Job drawing, mm, ordinate dimensions from the low corner. One solid piece. Give positions to 0.01 mm unless a question says otherwise; leave off trailing zeros. Loops run counter-clockwise (first coordinate to the right, second up) from the corner with the lowest first, then second, coordinate; pieces in that order, holes last. Notation, with made-up numbers: M 16,-6 L 29,-6 A20 cw 29,8 Z; hole C 14.25,54 d2. An arc over 180 degrees is marked long. Answer in a Markdown table with one row per item.
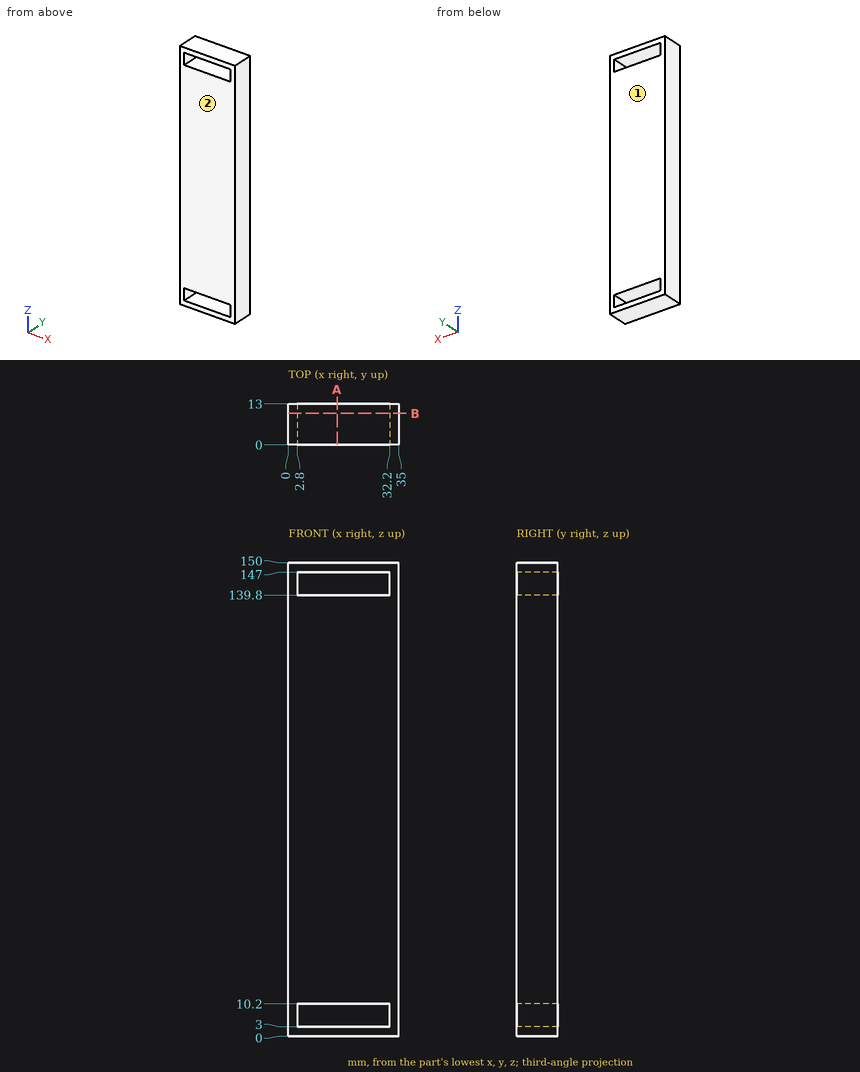
(1) Pull direction Y, two halves, no side cores. Call the marked faces 1 and 2: +Y half, -Y half, draft (parallel to the pull), parting line (faces both ways), or undercut.
Recorded:
| item | result |
|---|---|
| face 1 | +Y half |
| face 2 | -Y half |
(2) Drill centre lines: line 1 along Z through (x, y) = (9.5, 3.5); line 2 along X through (y, z) = (11, 9). Where is each one in solid material? Low to high.
Recorded:
| item | result |
|---|---|
| line 1 | z = 0 to 3, 10.2 to 139.8, 147 to 150 |
| line 2 | x = 0 to 2.8, 32.2 to 35 |
(3) Saw through at A-A (x = 15.5). Write the cut outline in (y, z).
Recorded:
| item | result |
|---|---|
| outline | M 0,0 L 13,0 L 13,3 L 0,3 Z; M 0,10.2 L 13,10.2 L 13,139.8 L 0,139.8 Z; M 0,147 L 13,147 L 13,150 L 0,150 Z |
(4) Pin check, flat tip, straight feed: pin 1 Ø2 at (x, y) = (21.5, 4) entering from -Z. Stop position of the tip, or through.
Recorded:
| item | result |
|---|---|
| pin 1 | stops at z = 0 |
(5) Saw through at B-B (y = 10). Write the cut outline in (x, z), plus the area to 3 significant figures.
Recorded:
| item | result |
|---|---|
| outline | M 0,0 L 35,0 L 35,150 L 0,150 Z; hole M 2.8,3 L 32.2,3 L 32.2,10.2 L 2.8,10.2 Z; hole M 2.8,139.8 L 32.2,139.8 L 32.2,147 L 2.8,147 Z |
| area | 4,830 mm^2 |
